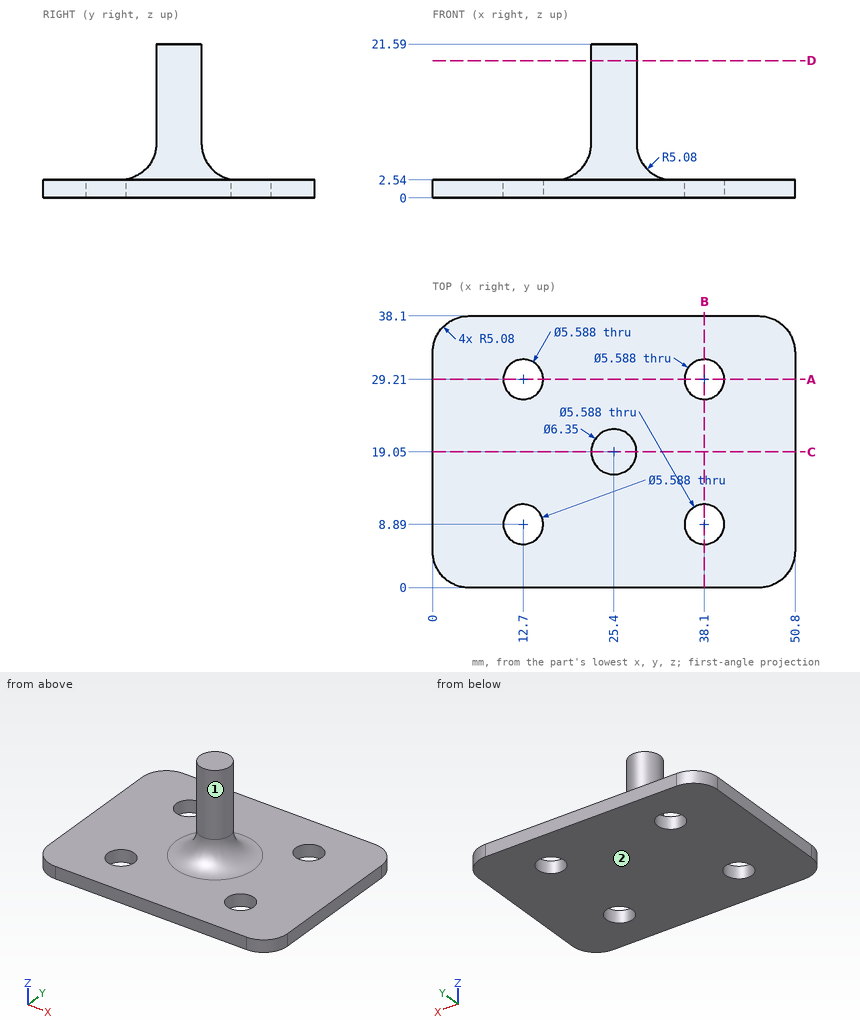
Geometry: see drawing. Coordinates: mm, zero at the bounding-box minimum. A direction names the side the tool comes from. Give positions to 0.01 mm unless a question says otherwise; leave off trailing zeros. Write each loop counter-clockwise with the first axis right and the second up, starting at its lowest first coordinate (ties: lowest second). Pieces come first, ordered by that corner, then holes. Notation, with made-up numbers: (51, -14) - (81, -14) arc R20 ccw to (81, 2) - close; hole circle Ø7 at (52.25, 75). An arc over 180 degrees is marked (long way). Return JSON: item names as keys, results as strings. Group by question number.
1) Line query: line 1 (Y direction, x = 38.1, z = 1.55); line 2 (Z direction, x = 6.5, y = 3.5); line 3 (Z direction, x = 31, y = 23). Output: solid intervals per line, ascending.
2) First-contact query: P1, Ø7.5, axis at x = 38.1, y = 29.21, coming from the +Z side; P2, Ø19, axis at x = 13.5, y = 13, coming from the +Z side; P3, Ø10, axis at x = 22.5, z = 18.5, coming from the -Y side (3 decimals); P4, Ø3.5, axis at x = 12.7, y = 8.89, coming from the -Z side. Flat tips, straight axial feed; report the tip coordinate or a pass-through.
3) Section C-C on y = 19.05. Return the cut outline in (x, z) (3 decimals).
4) Section B-B on x = 38.1. Return the cut outline in (y, z).
5) Set-up query: the marked faces 1 and 2. Return all of +Z, -Z, +X, -X, +Y, -Y with unobstructed straight access to the full face (end or side cutting, diameter ignored); none if empty.
6) Section A-A on y = 29.21. Return the cut outline in (x, z), plus the area to 3 significant figures.
7) Section D-D on z = 19.25. Return the cut outline in (x, y) (3 decimals).
Filled in:
{
 "1": {"line 1": "y = 0 to 6.1, 11.68 to 26.42, 32 to 38.1", "line 2": "z = 0 to 2.54", "line 3": "z = 0 to 2.74"},
 "2": {"P1": "stops at z = 2.54", "P2": "stops at z = 5.09", "P3": "stops at y = 15.875", "P4": "passes through"},
 "3": {"outline": "(0, 0) - (50.8, 0) - (50.8, 2.54) - (33.655, 2.54) arc R5.08 cw to (28.575, 7.62) - (28.575, 21.59) - (22.225, 21.59) - (22.225, 7.62) arc R5.08 cw to (17.145, 2.54) - (0, 2.54) - close"},
 "4": {"outline": "(0, 0) - (6.1, 0) - (6.1, 2.54) - (0, 2.54) - close; (11.68, 0) - (26.42, 0) - (26.42, 2.54) - (11.68, 2.54) - close; (32, 0) - (38.1, 0) - (38.1, 2.54) - (32, 2.54) - close"},
 "5": {"face 1": "+Z", "face 2": "-Z, +X, -X, +Y, -Y"},
 "6": {"outline": "(0, 0) - (9.91, 0) - (9.91, 2.54) - (0, 2.54) - close; (15.49, 0) - (35.31, 0) - (35.31, 2.54) - (15.49, 2.54) - close; (40.89, 0) - (50.8, 0) - (50.8, 2.54) - (40.89, 2.54) - close", "area": "101 mm^2"},
 "7": {"outline": "circle Ø6.35 at (25.4, 19.05)"}
}
